from build123d import *

# Parameters (mm, degrees)
BOSS_EXTRUDE1_DEPTH     = 12.7
SKETCH4_W               = 6.35
SKETCH4_H               = 2.9464
CUT_EXTRUDE1_DEPTH      = 19.020830121
LPATTERN1_COUNT         = 6
LPATTERN1_PITCH         = 12.7
CUT_EXTRUDE3_DEPTH      = 19.020830121
CUT_EXTRUDE3_DEPTH_BACK = 19.020830121
SKETCH9_R               = 1.8034


with BuildPart() as part:
    # Sketch3 → Boss-Extrude1 (new, symmetric)
    with BuildSketch(Plane(origin=(0, 0, 0), x_dir=(0, 0, -1), z_dir=(1, 0, 0))):
        with BuildLine():
            Line((0, -1.4732), (-12.7, -1.4732))
            Line((-12.7, -1.4732), (-12.7, -0.8382))
            Line((-12.7, -0.8382), (0, -0.8382))
            ThreePointArc((0, -0.8382), (0.421388638, 0.724576328), (-0.728533124, -0.414510226))
            Line((-0.728533124, -0.414510226), (-1.280452157, -0.728533124))
            ThreePointArc((-1.280452157, -0.728533124), (0.740622455, 1.273497789), (0, -1.4732))
        make_face()
    extrude(amount=BOSS_EXTRUDE1_DEPTH, both=True)

    # Sketch4 → Cut-Extrude1 (cut, symmetric)
    with BuildSketch(Plane(origin=(0, 0, 0), x_dir=(1, 0, 0), z_dir=(0, 1, 0))):
        with Locations((-3.175, 0)):
            Rectangle(SKETCH4_W, SKETCH4_H)
    cut_extrude1 = extrude(amount=CUT_EXTRUDE1_DEPTH, both=True, mode=Mode.SUBTRACT)

    # LPattern1: Cut-Extrude1 ×6
    with Locations(*[(i * LPATTERN1_PITCH, 0, 0) for i in range(1, LPATTERN1_COUNT)]):
        add(cut_extrude1, mode=Mode.SUBTRACT)

    # Cut-Extrude2 cone 1 section (through the dimple's axis) → Cut-Extrude2 (revolve, cut)
    with BuildSketch(Plane(origin=(7.9502, -0.8382, 7.5438), x_dir=(0, 0, 1), z_dir=(1, 0, 0))):
        Polygon((0, 0), (2.3114, 0), (0, 2.3114), align=None)
    revolve(axis=Axis((7.9502, -0.8382, 7.5438), (0, -1, 0)), mode=Mode.SUBTRACT)

    # Cut-Extrude2 cone 2 section (through the dimple's axis) → Cut-Extrude2 cone 2 (revolve, cut)
    with BuildSketch(Plane(origin=(-7.9248, -0.8382, 7.5438), x_dir=(0, 0, 1), z_dir=(1, 0, 0))):
        Polygon((0, 0), (2.3114, 0), (0, 2.3114), align=None)
    revolve(axis=Axis((-7.9248, -0.8382, 7.5438), (0, -1, 0)), mode=Mode.SUBTRACT)

    # Sketch9 → Cut-Extrude3 (cut, two sides: drawn at the far end of the back side and taken through both)
    with BuildSketch(Plane(origin=(0, 0, 0), x_dir=(1, 0, 0), z_dir=(0, 1, 0)).offset(-CUT_EXTRUDE3_DEPTH_BACK)):
        with Locations(Location((7.9502, -7.5438, 0), (0, 0, 270))):
            Circle(SKETCH9_R)
        with Locations(Location((-7.9248, -7.5438, 0), (0, 0, 270))):
            Circle(SKETCH9_R)
    extrude(amount=CUT_EXTRUDE3_DEPTH + CUT_EXTRUDE3_DEPTH_BACK, mode=Mode.SUBTRACT)


solid = part.part
Can you work these out from the model? Positions are in its coordinate system, mm. A direction names the side the tool comes from. Coordinates: 2 decimals unless noted, no trailing zeros. Order: outer loops, then holes, each group sorted by start corner. A loop starts at its lowest first (then second) coordinate and runs counter-clockwise, first axis right, second up. Notation, with made-up numbers: M 88,26 L 102,26 A15 cw 102,45 Z; hole C -32,-24.75 d9. An arc over 180 degrees is marked long. Answer as CSV lines item,"result".
(1) Suppose I cut it at A-A on y = 0. Please give me the cut outline in (x, z), plus the area to 3 significant figures.
Geometry check:
outline,"M -12.7,-1.47 L -6.35,-1.47 L -6.35,-0.84 L -12.7,-0.84 Z; M -12.7,0.84 L -6.35,0.84 L -6.35,1.47 L -12.7,1.47 Z; M 0,-1.47 L 6.35,-1.47 L 6.35,-0.84 L 0,-0.84 Z; M 0,0.84 L 6.35,0.84 L 6.35,1.47 L 0,1.47 Z"
area,"16.1 mm^2"
(2) Suppose I cut it at B-B on x = -4.75. Please give me the cut outline in (y, z).
Geometry check:
outline,"M -1.47,1.47 L -0.84,1.47 L -0.84,12.7 L -1.47,12.7 Z"
(3) Please list where these lines run through material, in increasing order: L1, parallel to Y at x = 2.75, z = 0; L2, parallel to X at y = -1.3, z = 6.25; L3, parallel to X at y = -1.3, z = 7.75.
Geometry check:
L1,"-1.47 to -0.84, 0.84 to 1.47"
L2,"-12.7 to -9.25, -6.6 to 6.63, 9.27 to 12.7"
L3,"-12.7 to -9.76, -6.09 to 6.11, 9.79 to 12.7"
(4) On a 3-axis mill with a long thin cutter (end or side, diameter ignored), from which of +Z, -Z, +X, -X, +Y, -Y can I reach the whole of each face in a straight line? I mean faces 4 (the flat face through (0, -1, 0)), 5 (the cylindrical face through (-9.481, 0.709, -0.448)). Say none if no direction works.
Geometry check:
face 4,"-Z, +Y, -Y"
face 5,"+X, -X"
(5) Suppose I cut it at D-D on x = 2. Please give me the cut outline in (y, z).
Geometry check:
outline,"M -1.47,0 A1.47 ccw long -0.73,1.28 L -0.41,0.73 A0.84 cw long -0.84,0 L -0.84,12.7 L -1.47,12.7 Z"
(6) Suppose I cut it at C-C on z = 7.75. Count the separate pieces of the cut face and the enclosed holes in it, plus the area to 3 significant figures.
Geometry check:
separate pieces,"3"
enclosed holes,"0"
area,"11.1 mm^2"
(7) I'm going to push flat-ended pins straight in: pin 1 (0.5 mm diameter, centred on x = 10.5, y = -1, fed in from -Z); pin 2 (5 mm diameter, centred on x = 5, z = 8, fed in from +Y). Where does each tip first touch, or does it pass through?
Geometry check:
pin 1,"z = 1.47"
pin 2,"y = -0.84"
(8) If we mould it in two halves opening along Z, with no side actions, what happens to faces 1 (the cylindrical face through (-9.48, 1.3, -0.69)), 2 (the flat face through (6.35, -1, 0)), 3 (the cylindrical face through (3.219, 0.709, -0.448))? For each: released by +Z, released by -Z, zero draft, split by the parting line, or undercut.
Geometry check:
face 1,"split by the parting line"
face 2,"zero draft"
face 3,"undercut"
